Part model, mm, in its own coordinate system. Face numbers are marked on the shaded views. Round coordinates to 2 decimals unless told otherwise and drop trailing zeros. Write each loop counter-clockwise with the first axis right and the second up, starting at its lowest first coordinate (ties: lowest second). Pieces come first, ordered by that corner, then holes.
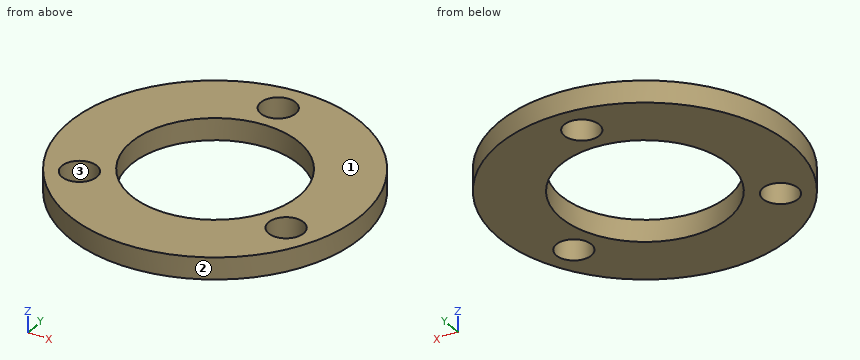
```python
from build123d import *

# Parameters (mm, degrees)
SKETCH2_R           = 20
SKETCH2_R_2         = 2.4
SKETCH2_R_3         = 11.5
BOSS_EXTRUDE1_DEPTH = 3


with BuildPart() as part:
    # Sketch2 → Boss-Extrude1 (new body)
    with BuildSketch(Plane.XY):
        Circle(SKETCH2_R)
        with Locations((-13.184775653, -8.660341037)):
            Circle(SKETCH2_R_2, mode=Mode.SUBTRACT)
        with Locations((13.958150794, -7.065513271)):
            Circle(SKETCH2_R_2, mode=Mode.SUBTRACT)
        Circle(SKETCH2_R_3, mode=Mode.SUBTRACT)
        with Locations((-0.89182915, 15.582825039)):
            Circle(SKETCH2_R_2, mode=Mode.SUBTRACT)
    extrude(amount=BOSS_EXTRUDE1_DEPTH)


solid = part.part
```
Q1. Cut at A-A on y = 0. Write the cut outline in (x, z).
Values follow:
outline: (-20, 0) - (-11.5, 0) - (-11.5, 3) - (-20, 3) - close; (11.5, 0) - (20, 0) - (20, 3) - (11.5, 3) - close
Q2. Cut at C-C on z = 1. Write the cut outline in (x, y), plus the area to 3 significant figures.
Values follow:
outline: circle Ø40 at (0, 0); hole circle Ø4.8 at (-13.18, -8.66); hole circle Ø23 at (0, 0); hole circle Ø4.8 at (-0.89, 15.58); hole circle Ø4.8 at (13.96, -7.07)
area: 787 mm2
Q3. Mould opens along X. For the marked faces 1, 2 and 3 say: +X half, -X half, draft (parallel to the pull), parting line (faces both ways), or undercut.
Values follow:
face 1: draft
face 2: parting line
face 3: undercut
Q4. Cut at B-B on x = -1.5. Write the cut outline in (y, z), plus the area to 3 significant figures.
Values follow:
outline: (-19.94, 0) - (-11.4, 0) - (-11.4, 3) - (-19.94, 3) - close; (11.4, 0) - (13.26, 0) - (13.26, 3) - (11.4, 3) - close; (17.9, 0) - (19.94, 0) - (19.94, 3) - (17.9, 3) - close
area: 37.3 mm2
Q5. Wall check: L1, parallel to X at y = -5, z = 2.55; L2, parallel to X at y = -8, z = 2.1; L3, parallel to Y at x = -2, z = 1.25. Give the ranges that are in metal, low to high.
Values follow:
L1: x = -19.36 to -10.36, 10.36 to 12.74, 15.18 to 19.36
L2: x = -18.33 to -15.49, -10.88 to -8.26, 8.26 to 11.75, 16.17 to 18.33
L3: y = -19.9 to -11.32, 11.32 to 13.45, 17.71 to 19.9
Q6. Cut at D-D on x = 4. Write the cut outline in (y, z).
Values follow:
outline: (-19.6, 0) - (-10.78, 0) - (-10.78, 3) - (-19.6, 3) - close; (10.78, 0) - (19.6, 0) - (19.6, 3) - (10.78, 3) - close
Q7. Drop flat-ended pins along their axis: pin 1 (4.5 mm diameter, centred on x = 13.96, y = -7.07, fed in from +Z); pin 2 (8 mm diameter, centred on x = 8, y = -1.5, fed in from +Z). Give the stop position or say it passes through.
Values follow:
pin 1: passes through
pin 2: stops at z = 3
